Here's the drawing with two shaded views (mm, measured from the low corner). I have some questions. Round coordinates to 2 decimals unless told otherwise and drop trailing zeros. Write each loop counter-clockwise with the first axis right and the second up, starting at its lowest first coordinate (ties: lowest second). Pieces come first, ordered by that corner, then holes. Notation, with made-up numbers: M 62,63 L 86,63 A23 cw 86,88 Z; hole C 27.5,31 d11. An arc over 180 degrees is marked long. Use one line per item in the form item = value. Start each with the question number.
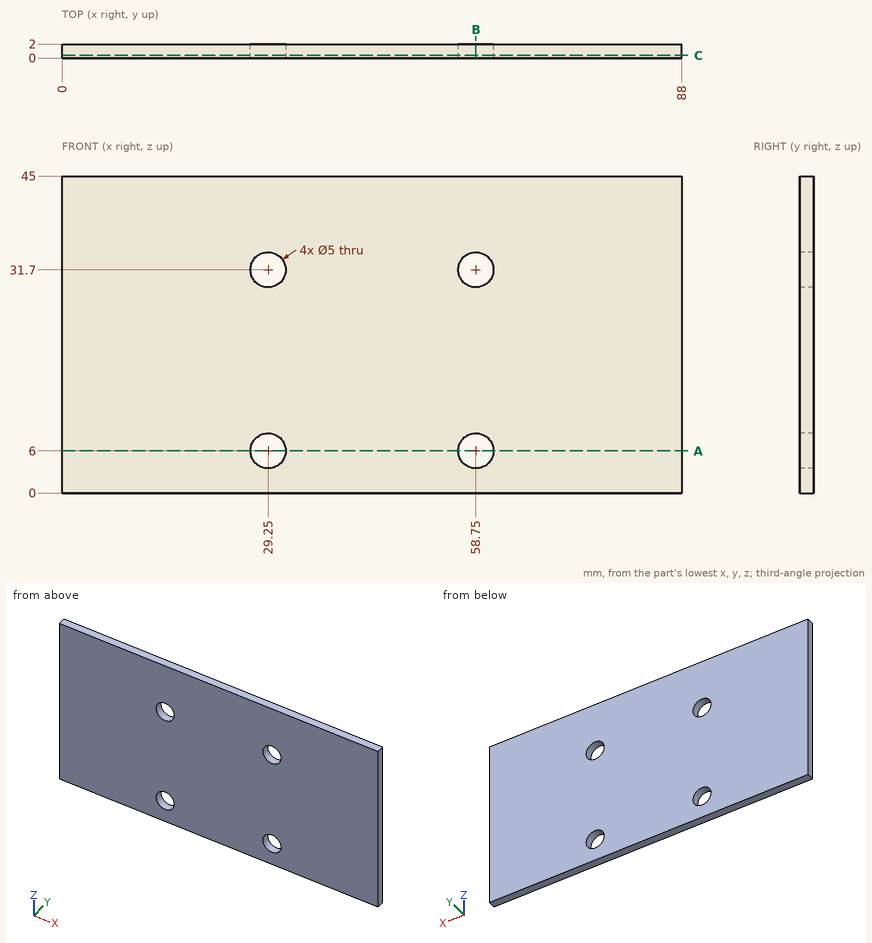
1. Please list where these lines run through material, in increasing order: line 1 along Z through (x, y) = (29.25, 0.55); line 2 along X through (y, z) = (1.5, 32); line 3 along Z through (x, y) = (57, 0.15).
2. If we section it at B-B (x = 58.75): List the corners of the cut face in (y, z) for me, and give its area (3 significant figures).
3. If we section it at C-C (y = 0.4): List the corners of the cut face in (x, z) for me, and give its area (3 significant figures).
4. Will this pin go through, and if not, where does the flat tip stop? pin 1 (8 mm diameter, centred on x = 58.75, z = 6, fed in from -Y).
5. If we section it at A-A (z = 6): List the corners of the cut face in (x, y) for me, and give its area (3 significant figures).
Model answer:
q1.line_1 = 0 to 3.5, 8.5 to 29.2, 34.2 to 45
q1.line_2 = 0 to 26.77, 31.73 to 56.27, 61.23 to 88
q1.line_3 = 0 to 4.21, 7.79 to 29.91, 33.49 to 45
q2.outline = M 0,0 L 2,0 L 2,3.5 L 0,3.5 Z; M 0,8.5 L 2,8.5 L 2,29.2 L 0,29.2 Z; M 0,34.2 L 2,34.2 L 2,45 L 0,45 Z
q2.area = 70.0 mm2
q3.outline = M 0,0 L 88,0 L 88,45 L 0,45 Z; hole C 29.25,6 d5; hole C 29.25,31.7 d5; hole C 58.75,6 d5; hole C 58.75,31.7 d5
q3.area = 3,880 mm2
q4.pin_1 = 0
q5.outline = M 0,0 L 26.75,0 L 26.75,2 L 0,2 Z; M 31.75,0 L 56.25,0 L 56.25,2 L 31.75,2 Z; M 61.25,0 L 88,0 L 88,2 L 61.25,2 Z
q5.area = 156 mm2
